```python
from build123d import *

# Parameters (mm, degrees)
F0_W     = 134.112
F0_H     = 134.112
F1_DEPTH = 25.4
F2_DEPTH = 2.794
F0_W_2   = 1.9812
F0_H_2   = 50.8
F3_DEPTH = 190.5
F4_DEPTH = 25.4
F5_R     = 8.89
F6_DEPTH = 143.6634


# Not quite as in the source:
# - a feature of the source that left no trace in its solid (it failed there, or was rolled back) is left out


with BuildPart() as f1:
    # F0 (on Top) → F1 (new body)
    with BuildSketch(Plane.XY):
        Polygon((0, 44.45), (0, 0), (139.7, 0), (139.7, 44.45), (139.7, 95.25), (139.7, 139.7), (0, 139.7), (0, 95.25), align=None)
        with Locations((69.85, 69.85)):
            Rectangle(F0_W, F0_H, mode=Mode.SUBTRACT)
    extrude(amount=-F1_DEPTH)

    # F0 (on Top) → F2 (join)
    with BuildSketch(Plane.XY):
        with Locations((69.85, 69.85)):
            Rectangle(F0_W, F0_H)
    extrude(amount=-F2_DEPTH)

    # F0 (on Top) → F3 (join)
    with BuildSketch(Plane.XY):
        with Locations((-0.9906, 69.85)):
            Rectangle(F0_W_2, F0_H_2)
        with Locations((140.6906, 69.85)):
            Rectangle(F0_W_2, F0_H_2)
    extrude(amount=F3_DEPTH)

    # F0 (on Top) → F4 (join)
    with BuildSketch(Plane.XY):
        with Locations((-0.9906, 69.85)):
            Rectangle(F0_W_2, F0_H_2)
        with Locations((140.6906, 69.85)):
            Rectangle(F0_W_2, F0_H_2)
    extrude(amount=-F4_DEPTH)

    # F5 (on face) → F6 (cut, through all)
    with BuildSketch(Plane.YZ.offset(141.6812)):
        with Locations((69.85, 165.1)):
            Circle(F5_R)
        with Locations((69.85, 101.6)):
            Circle(F5_R)
    extrude(amount=-F6_DEPTH, mode=Mode.SUBTRACT)


solid = f1.part
```
Work out the finished part from the listing and answer in its coordinate system (mm). A direction names the side the tool comes from. Coordinates: 2 decimals unless noted, no trailing zeros. Write each loop counter-clockwise with the first axis right and the second up, starting at its lowest first coordinate (ties: lowest second). Pieces come first, ordered by that corner, then holes.
Q1. Each of these flat-tipped pins is pushed along its axis until it touches: pin 1 Ø1 at (x, z) = (-0.5, 123.5) entering from -Y; pin 2 Ø1.5 at (y, z) = (102.5, -1) entering from +X; pin 3 Ø2 at (x, z) = (141, 73) entering from +Y. Where does it stop, or does it pass through?
Q2. Determine the mould class of faces 1 (the face through (140.7, 67.92, 156.42)), 2 (the face through (0, 23, -13)), 3 (the face through (139.7, 117, -13)), 4 (the face through (0, 75, 94)) for opening direction X: released by +X, released by -X, zero draft, split by the parting line, or undercut.
Q3. A cutting plane is placed at A-A, the plane y = 69.85. Give the vertices of the cut face in (x, z), then the cut area to 3 significant figures.
Q4. A cutting plane is placed at B-B, the plane z = 84. Give the vertices of the cut face in (x, y), then the cut area to 3 significant figures.
Q5. Find the intervals of material crossed by line 1 (Z direction, x = 140.45, y = 69.85); line 2 (X direction, y = 46, z = 37); line 3 (Y direction, x = -1, z = 101), in increasing order.
Q6. A cutting plane is placed at C-C, the plane y = 48. Give the vertices of the cut face in (x, z).
Q7. Which of the six approach directions +Z, -Z, +X, -X, +Y, -Y give full straight-line access (tool end or side, diameter ignored) to faces 5 (the face through (69, 71, 0)), 6 (the face through (2.794, 69, -14)), 7 (the face through (139.7, 22, -13)), 8 (the face through (0, 118, -13)), 9 (the face through (69.5, 137.4, -25.4))?
Q8. A cutting plane is placed at D-D, the plane x = 63. Give the vertices of the cut face in (y, z).
Findings below:
1. pin 1: stops at y = 44.45
1. pin 2: stops at x = 139.7
1. pin 3: stops at y = 95.25
2. face 1: zero draft
2. face 2: released by -X
2. face 3: released by +X
2. face 4: undercut
3. outline: (-1.98, -25.4) - (2.79, -25.4) - (2.79, -2.79) - (136.91, -2.79) - (136.91, -25.4) - (141.68, -25.4) - (141.68, 92.71) - (139.7, 92.71) - (139.7, 0) - (0, 0) - (0, 92.71) - (-1.98, 92.71) - close; (-1.98, 110.49) - (0, 110.49) - (0, 156.21) - (-1.98, 156.21) - close; (-1.98, 173.99) - (0, 173.99) - (0, 190.5) - (-1.98, 190.5) - close; (139.7, 110.49) - (141.68, 110.49) - (141.68, 156.21) - (139.7, 156.21) - close; (139.7, 173.99) - (141.68, 173.99) - (141.68, 190.5) - (139.7, 190.5) - close
3. area: 1,230 mm2
4. outline: (-1.98, 44.45) - (0, 44.45) - (0, 95.25) - (-1.98, 95.25) - close; (139.7, 44.45) - (141.68, 44.45) - (141.68, 95.25) - (139.7, 95.25) - close
4. area: 201 mm2
5. line 1: z = -25.4 to 92.71, 110.49 to 156.21, 173.99 to 190.5
5. line 2: x = -1.98 to 0, 139.7 to 141.68
5. line 3: y = 44.45 to 60.98, 78.72 to 95.25
6. outline: (-1.98, -25.4) - (2.79, -25.4) - (2.79, -2.79) - (136.91, -2.79) - (136.91, -25.4) - (141.68, -25.4) - (141.68, 190.5) - (139.7, 190.5) - (139.7, 0) - (0, 0) - (0, 190.5) - (-1.98, 190.5) - close
7. face 5: +Z, +Y, -Y
7. face 6: -Z
7. face 7: +Z, -Z, +X, -Y
7. face 8: +Z, -Z, -X, +Y
7. face 9: -Z, +X, -X, +Y, -Y
8. outline: (0, -25.4) - (2.79, -25.4) - (2.79, -2.79) - (136.91, -2.79) - (136.91, -25.4) - (139.7, -25.4) - (139.7, 0) - (0, 0) - close
